Geometry check sheet. Reference: drawing and pictorial views, mm from the part's lowest x, y, z. Coordinates: 2 decimals unless noted, no trailing zeros. Write each loop counter-clockwise with the first axis right and the second up, starting at its lowest first coordinate (ties: lowest second). Pieces come first, ordered by that corner, then holes. Notation, with made-up numbers: (82.5, 51) - (130.5, 51) arc R17 cw to (130.5, 77) - close; hole circle Ø2 at (56.5, 83). An arc over 180 degrees is marked (long way). Use one line per item in the form item = value. Start each with the question number.
(1) Sectioned sample at C-C (y = 1.8). Record the cut outline in (x, z).
(2) Sectioned sample at D-D (x = 4.8). Record the cut outline in (y, z), and give its area (3 significant figures).
(3) Gauge pin test, flat ends, axial feed: pin 1 Ø1.8 at (x, z) = (3.5, 2.5) entering from +Y; pin 2 Ø1.5 at (x, y) = (3, 2) entering from +Z. Record the tip position at first contact, or that the pin passes through.
(4) Mould release check, pull along Z, two halves, no side actions. Record for the marked faces 1, 2 and 3: released by +Z, released by -Z, zero draft, split by the parting line, or undercut.
(5) Sectioned sample at B-B (x = 1.8). Record the cut outline in (y, z), and give its area (3 significant figures).
(6) Material ranges on line 1 (X direction, y = 1.2, z = 3); line 2 (X direction, y = 0.6, z = 3); line 3 (Y direction, x = 5.1, z = 1.5), recorded low to high. Write a range as [from, to].
(7) Sectioned sample at A-A (z = 3). Record the cut outline in (x, y).
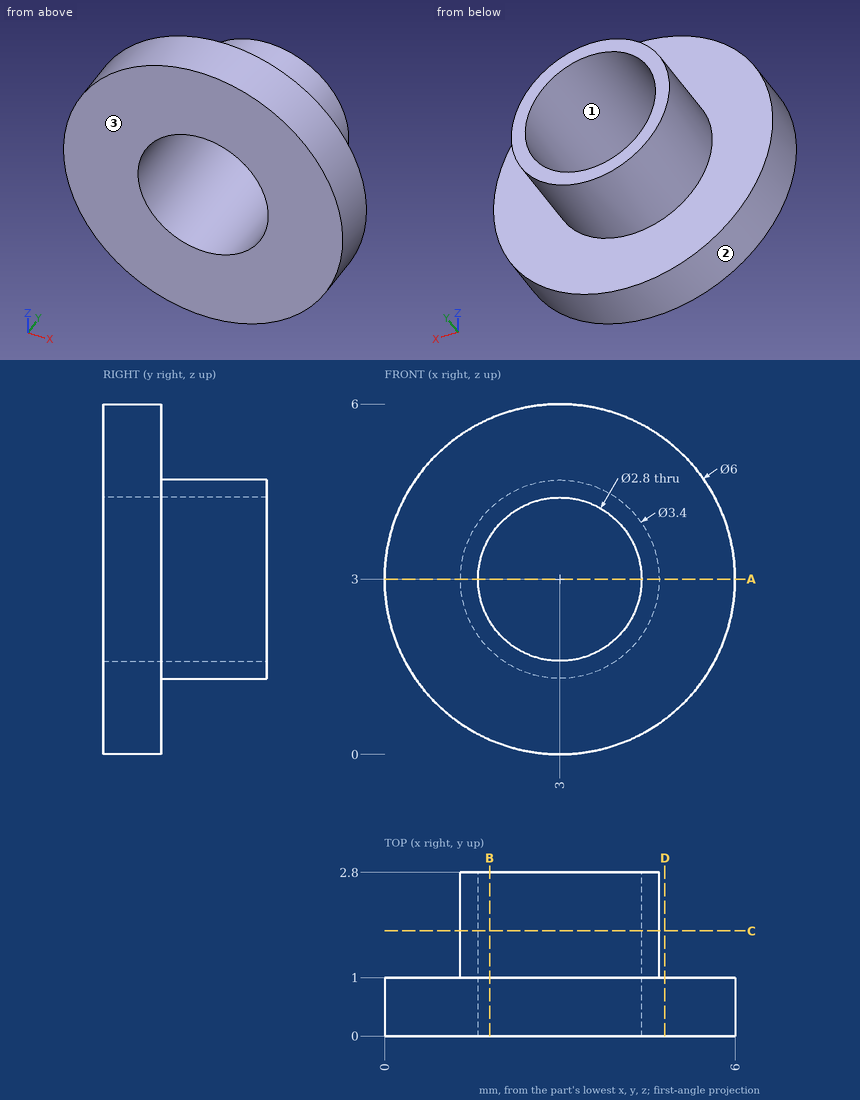
Answers below:
q1.outline = circle Ø3.4 at (3, 3); hole circle Ø2.8 at (3, 3)
q2.outline = (0, 0.6) - (1, 0.6) - (1, 5.4) - (0, 5.4) - close
q2.area = 4.80 mm2
q3.pin_1 = 2.8
q3.pin_2 = 4.7
q4.face_1 = undercut
q4.face_2 = split by the parting line
q4.face_3 = zero draft
q5.outline = (0, 0.25) - (1, 0.25) - (1, 1.8) - (2.8, 1.8) - (2.8, 2.28) - (0, 2.28) - close; (0, 3.72) - (2.8, 3.72) - (2.8, 4.2) - (1, 4.2) - (1, 5.75) - (0, 5.75) - close
q5.area = 5.80 mm2
q6.line_1 = [1.3, 1.6], [4.4, 4.7]
q6.line_2 = [0, 1.6], [4.4, 6]
q6.line_3 = [0, 1]
q7.outline = (0, 0) - (1.6, 0) - (1.6, 2.8) - (1.3, 2.8) - (1.3, 1) - (0, 1) - close; (4.4, 0) - (6, 0) - (6, 1) - (4.7, 1) - (4.7, 2.8) - (4.4, 2.8) - close
